from build123d import *

# Parameters (mm, degrees)
SKETCH1_R           = 9.5
BOSS_EXTRUDE1_DEPTH = 24
SKETCH2_R           = 4
CUT_EXTRUDE1_DEPTH  = 12
SKETCH3_R           = 2.5
CUT_EXTRUDE2_DEPTH  = 12


with BuildPart() as part:
    # Sketch1 → Boss-Extrude1 (new body)
    with BuildSketch(Plane(origin=(0, 0, 0), x_dir=(1, 0, 0), z_dir=(0, 1, 0))):
        Circle(SKETCH1_R)
    extrude(amount=BOSS_EXTRUDE1_DEPTH)

    # Sketch2 → Cut-Extrude1 (cut)
    with BuildSketch(Plane(origin=(0, 24, 0), x_dir=(1, 0, 0), z_dir=(0, 1, 0))):
        Circle(SKETCH2_R)
    extrude(amount=-CUT_EXTRUDE1_DEPTH, mode=Mode.SUBTRACT)

    # Sketch3 → Cut-Extrude2 (cut)
    with BuildSketch(Plane.XZ):
        Circle(SKETCH3_R)
    extrude(amount=-CUT_EXTRUDE2_DEPTH, mode=Mode.SUBTRACT)


solid = part.part
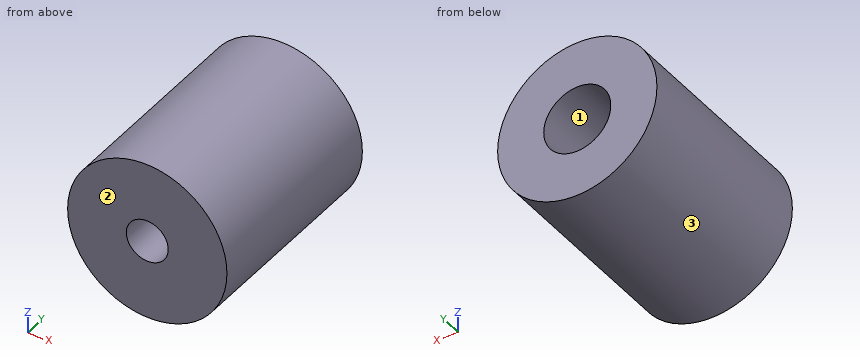
The listing builds one solid part. Answer for the finished solid, in the listing's coordinates (mm). Face numbers are marked on the shaded views. Round coordinates to 2 decimals unless told otherwise and drop trailing zeros. Write each loop counter-clockwise with the first axis right and the second up, starting at its lowest first coordinate (ties: lowest second). Pieces come first, ordered by that corner, then holes. Notation, with made-up numbers: M -36.5,65 L -18.5,65 A18 cw -18.5,85 Z; hole C -15,75 d8. An arc over 180 degrees is marked long. Write each question's results on one line, items separated by ' | '. Start each with the question number.
(1) The part is cut by section C-C, the plane y = 17. Write down the section's boundary in (x, z).
(2) The part is cut by section A-A, the plane z = 0. Write down the section's boundary in (x, y), and give its area (3 significant figures).
(3) The part is cut by section D-D, the plane x = -3. Write down the section's boundary in (y, z), and give its area (3 significant figures).
(4) The part is cut by section B-B, the plane x = 0. Write down the section's boundary in (y, z).
(5) Find the intervals of material crossed by line 1 (Z direction, x = 0, y = 15.25); line 2 (Z direction, x = 0, y = 3.5), in increasing order.
(6) Determine the mould class of the marked faces 1, 2 and 3 for opening direction Z: +Z half, -Z half, draft (parallel to the pull), parting line (faces both ways), or undercut.
(7) Each of these flat-tipped pins is pushed along its axis until it touches: P1, Ø4, axis at x = -7, y = 4, coming from the +Z side; P2, Ø8, axis at x = -6.5, y = 11, coming from the -Z side; P3, Ø4, axis at x = -5.5, y = 8.5, coming from the -Z side. Where does it stop, or does it pass through?
Worked answers:
1) outline: C 0,0 d19; hole C 0,0 d8
2) outline: M -9.5,0 L -2.5,0 L -2.5,12 L -4,12 L -4,24 L -9.5,24 Z; M 2.5,0 L 9.5,0 L 9.5,24 L 4,24 L 4,12 L 2.5,12 Z | area: 300 mm²
3) outline: M 0,-9.01 L 24,-9.01 L 24,-2.65 L 12,-2.65 L 12,2.65 L 24,2.65 L 24,9.01 L 0,9.01 Z | area: 369 mm²
4) outline: M 0,-9.5 L 24,-9.5 L 24,-4 L 12,-4 L 12,-2.5 L 0,-2.5 Z; M 0,2.5 L 12,2.5 L 12,4 L 24,4 L 24,9.5 L 0,9.5 Z
5) line 1: z = -9.5 to -4, 4 to 9.5 | line 2: z = -9.5 to -2.5, 2.5 to 9.5
6) face 1: undercut | face 2: draft | face 3: parting line
7) P1: stops at z = 8.08 | P2: stops at z = -9.17 | P3: stops at z = -8.83
